from build123d import *

# Parameters (mm, degrees)
F1_DEPTH  = 40
F4_DEPTH  = 62.5
F6_DEPTH  = 12.5
F8_DEPTH  = 25
F10_DEPTH = 5
F12_DEPTH = 15


# Not quite as in the source:
# - a pattern or mirror of a feature is missing from the dataset's text; its kind, count and spacing are read off the source's solid


with BuildPart() as f1:
    # F0 (on Right) → F1 (new body)
    with BuildSketch(Plane.YZ):
        Polygon((-57.0501919146, 0), (0, 0), (42.9498080854, 0), (42.9498080854, 10), (-57.0501919146, 10), align=None)
    extrude(amount=F1_DEPTH)

    # F3 (on offset) → F4 (join)
    with BuildSketch(Plane.YZ.offset(51.25)):
        Polygon((9.1779063212, 130.638949744), (30.4498080854, 10), (42.9498080854, 10), (21.6779063212, 130.638949744), align=None)
    extrude(amount=-F4_DEPTH)

    # F5 (on face) → F6 (join)
    with BuildSketch(Plane(origin=(0, 42.9498080854, 0), x_dir=(-1, 0, 0), z_dir=(0, 1, 0))):
        Polygon((11.25, 10), (0, 10), (0, 0), align=None)
        Polygon((-40, 0), (-40, 10), (-51.25, 10), align=None)
    extrude(amount=-F6_DEPTH)

    # F7 (on face) → F8 (join)
    with BuildSketch(Plane.XY.offset(10)):
        Polygon((15.9533534884, -42.2205627832), (6.2940952255, -39.6323723322), (5, -44.4620014636), (14.6592582629, -47.0501919146), align=None)
        Polygon((33.7059047745, -39.6323723322), (24.0466465116, -42.2205627832), (25.3407417371, -47.0501919146), (35, -44.4620014636), align=None)
    extrude(amount=F8_DEPTH)

    # F9 (on face) → F10 (join)
    with BuildSketch(Plane(origin=(-9.4864686499, -35.4039829857, 0), x_dir=(-0.9659258263, 0.2588190451, 0), z_dir=(0.2588190451, 0.9659258263, 0))):
        Polygon((-16.3372418936, 35), (-16.3372418936, 10), (0, 35), align=None)
    f10 = extrude(amount=-F10_DEPTH)

    # F10_copies: F10 across plane
    add(f10.mirror(Plane(origin=(20, 0, 0), x_dir=(0, 0, 1), z_dir=(1, 0, 0))))

    # F11 (on face) → F12 (cut)
    with BuildSketch(Plane.XY.offset(35)):
        Polygon((12.2791188742, -44.3418831268), (12.4861741103, -43.5691424657), (-10.0558705491, -37.5290198035), (-10.2629257852, -38.3017604645), align=None)
    f12 = extrude(amount=-F12_DEPTH, mode=Mode.SUBTRACT)

    # F12_copies: F12 across plane
    add(f12.mirror(Plane(origin=(20, 0, 0), x_dir=(0, 0, 1), z_dir=(1, 0, 0))), mode=Mode.SUBTRACT)


solid = f1.part
Here's how the part is built. I have some questions about the finished solid (model axes, mm). A direction names the side the tool comes from. Coordinates: 2 decimals unless noted, no trailing zeros. Write each loop counter-clockwise with the first axis right and the second up, starting at its lowest first coordinate (ties: lowest second). Pieces come first, ordered by that corner, then holes.
Item 1: I want a section at D-D on y = -17. Write out the boundary of the cut face in (x, z).
Item 2: On a 3-axis mill with a long thin cutter (end or side, diameter ignored), from which of +Z, -Z, +X, -X, +Y, -Y can I reach the whole of each face in a straight line? I mean faces 1 (the flat face through (20.438, 19.665, 71.164)), 2 (the flat face through (15.297, -44.669, 22.325)), 3 (the flat face through (34, -42, 20)), 4 (the flat face through (37.4, -40.6, 35)), 5 (the flat face through (41.98, -39.392, 22.325)). Say none if no direction works.
Item 3: I want a section at B-B on x = 47. Write out the boundary of the cut face in (y, z).
Item 4: I want a section at C-C on x = 18. Write out the boundary of the cut face in (y, z).
Item 5: Will these pins go through, and if not, where does the flat tip stop? pin 1 (5 mm diameter, centred on x = -7, z = 6.5, fed in from -Y); pin 2 (8 mm diameter, centred on x = 40, z = 75.5, fed in from -Y); pin 3 (1 mm diameter, centred on x = 11.5, z = 26.5, fed in from -Y); pin 4 (12 mm diameter, centred on x = 41, y = -4, fed in from -Z).
Item 6: I want a section at A-A on z = 23. Write out the boundary of the cut face in (x, y), and give its area (3 significant figures).
Item 7: If we mould it in two halves opening along Y, with no side actions, what happens to faces 6 (the flat face through (-11.25, 26, 71)), 7 (the flat face through (43, 30.45, 7)), 8 (the flat face through (36.65, -41.95, 27.61)), 9 (the flat face through (20, 42.95, 5))? For each: +Y half, -Y half, draft (parallel to the pull), parting line (faces both ways), or undercut.
Item 8: If I drill on line 1 (Y direction, x = -2.5, z = 31); line 2 (Z direction, x = 11.5, y = -32.5); line 3 (Z direction, x = 13, y = -46.5), over which ranges is the centre line in solid material (lowest first)?
Findings below:
1. outline: (0, 0) - (40, 0) - (40, 10) - (0, 10) - close
2. face 1: +X, -X
2. face 2: +Z, -Y
2. face 3: +Z
2. face 4: +Z, +X, -X, -Y
2. face 5: +X
3. outline: (-41.25, 29.01) - (-39.18, 29.83) - (-39.18, 35) - (-41.25, 35) - close; (-38.35, 30.16) - (-36.07, 31.06) - (-36.07, 35) - (-38.35, 35) - close; (9.18, 130.64) - (30.45, 10) - (30.45, 6.22) - (42.95, 6.22) - (42.95, 10) - (21.68, 130.64) - close
4. outline: (-57.05, 0) - (42.95, 0) - (42.95, 10) - (21.68, 130.64) - (9.18, 130.64) - (30.45, 10) - (-57.05, 10) - close
5. pin 1: stops at y = 30.45
5. pin 2: stops at y = 18.2
5. pin 3: stops at y = -46.34
5. pin 4: stops at z = 0
6. outline: (-11.25, 28.16) - (51.25, 28.16) - (51.25, 40.66) - (-11.25, 40.66) - close; (-3.21, -42.26) - (14.66, -47.05) - (15.95, -42.22) - (-1.91, -37.43) - (-2.48, -39.56) - (12.49, -43.57) - (12.28, -44.34) - (-2.69, -40.33) - close; (24.05, -42.22) - (25.34, -47.05) - (43.21, -42.26) - (42.69, -40.33) - (27.72, -44.34) - (27.51, -43.57) - (42.48, -39.56) - (41.91, -37.43) - close
6. area: 941 mm2
7. face 6: draft
7. face 7: -Y half
7. face 8: undercut
7. face 9: +Y half
8. line 1: y = -42.45 to -40.38, -39.55 to -37.28, 26.75 to 39.25
8. line 2: z = 0 to 10
8. line 3: z = 0 to 35
